Autodesk Inventor part; units mm, degrees
ref_plane "YZ Plane" through (0, 0, 0) normal (1, 0, 0) x (0, 1, 0)
ref_plane "XZ Plane" through (0, 0, 0) normal (0, 1, 0) x (-1, 0, 0)
ref_plane "XY Plane" through (0, 0, 0) normal (0, 0, 1) x (1, 0, 0)
sketch "Sketch1" plane through (0, 0, 0) normal (0, 0, 1) x (1, 0, 0)
  line L0 (965.2, 50.7572) -> (1117.6, 50.7572)
  line L1 (1117.6, 50.7572) -> (1117.6, -0.0428)
  line L2 (1117.6, -0.0428) -> (0, -0.0428)
  line L3 (0, -0.0428) -> (0, 25.3572)
  line L4 (0, 25.3572) -> (965.2, 50.7572)
  point P0 (0, 0)
extrude "Extrusion1" add sketch "Sketch1" along normal blind 19.05
properties part number "nd-a"
Geometry check sheet. Reference: the model listing, model coordinates, mm. Coordinates: 2 decimals unless noted, no trailing zeros. Order: outer loops, then holes, each group sorted by start corner. A loop starts at its lowest first (then second) coordinate and runs counter-clockwise, first axis right, second up. Notation, with made-up numbers: (62.25, 36.25) - (90.25, 36.25) arc R15 ccw to (90.25, 40.25) - close; hole circle Ø2 at (28.25, 27). An arc over 180 degrees is marked (long way). Answer as a JSON object with one key per item and string values. Group by question number.
Item 1: Sectioned sample at B-B, the plane x = 267.5. Record the cut outline in (y, z), and give its area (3 significant figures).
Item 2: Sectioned sample at A-A, the plane z = 9. Record the cut outline in (x, y).
Item 3: Sectioned sample at C-C, the plane y = 41. Record the cut outline in (x, z), and give its area (3 significant figures).
Item 4: Depth check by flat-ended pin: pin 1 Ø2 at (x, z) = (510, 8.5) entering from +Y; pin 2 Ø4 at (x, z) = (441.5, 15) entering from +Y; pin 3 Ø2 at (x, z) = (326, 11) entering from +Y. Enter the tip coordinate at first touch or a pass-through.
Item 5: Scan lines: probe 1 along Y at (x, z) = (115, 4.25); probe 2 along Y at (x, z) = (392.5, 13.25). Record each from-to range of solid material in increasing order.
Resolved:
{
 "1": {"outline": "(-0.04, 0) - (32.4, 0) - (32.4, 19.05) - (-0.04, 19.05) - close", "area": "618 mm^2"},
 "2": {"outline": "(0, -0.04) - (1117.6, -0.04) - (1117.6, 50.76) - (965.2, 50.76) - (0, 25.36) - close"},
 "3": {"outline": "(594.43, 0) - (1117.6, 0) - (1117.6, 19.05) - (594.43, 19.05) - close", "area": "9,970 mm^2"},
 "4": {"pin 1": "y = 38.8", "pin 2": "y = 37.03", "pin 3": "y = 33.96"},
 "5": {"probe 1": "-0.04 to 28.38", "probe 2": "-0.04 to 35.69"}
}
